Can you work these out from the model? Positions are in its coordinate system, mm. Face numbers are marked on the shaded views. A direction names the side the tool comes from. Coordinates: 2 decimals unless noted, no trailing zeros. Order: outer loops, then holes, each group sorted by start corner. A loop starts at its lowest first (then second) coordinate and runs counter-clockwise, first axis right, second up. Notation, with made-up numbers: (-3, 17) -> (38, 17) arc R12 ccw to (38, 25) -> close; hole circle Ø7 at (62.5, 6.25). An arc over 180 degrees is marked (long way). Answer as a JSON object with one key per item and string values. Group by question number.
(1) If we mould it in two halves opening along X, with no side actions, what happens to the marked faces 1, 2 and 3? For each: pulls with the +X half, pulls with the -X half, needs draft (parallel to the pull), parting line crosses it, or undercut.
(2) I want a section at C-C, the plane z = 8.5. List the corners of the cut face in (x, y) for me.
(3) For pin 1 (4.5 mm diameter, centred on y = 38.58, z = 7.34, fed in from -X); pin 2 (17.5 mm diameter, centred on x = 21.5, z = 24.5, fed in from +Y), each with a flat end and sliding along its axis, tell me the tip position at first contact or that it passes through.
(4) I need wall thicknesses on line 1 (Z direction, x = 20, y = 4); line 2 (X direction, y = 19, z = 19); line 3 (Z direction, x = 19.5, y = 4). Which ranges of each line are inside material? Lowest first, please.
(5) I want a section at D-D, the plane z = 28.5. List the corners of the cut face in (x, y) for me.
(6) Which directions (+Z, -Z, +X, -X, +Y, -Y) give clear straight access to the entire face, cutting with the end or side of a thin tool? Please do the marked faces 4 and 5.
(7) I want a section at A-A, the plane y = 12. List the corners of the cut face in (x, z) for me, plus the area to 3 significant figures.
(8) I want a section at B-B, the plane x = 20. List the corners of the cut face in (y, z) for me.
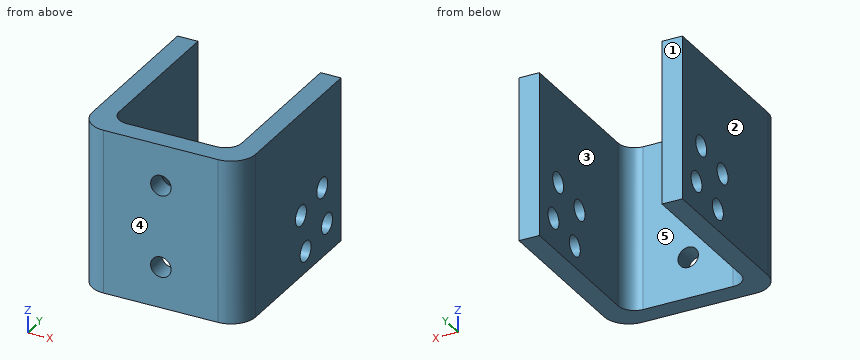
from build123d import *

# Parameters (mm, degrees)
RESSALTO_EXTRUS_O1_DEPTH = 40
FILETE1_R                = 6
ESBO_O3_R                = 2.5
CORTE_EXTRUS_O1_DEPTH    = 60
FILETE2_R                = 4
ESBO_O6_R                = 2.5
CORTE_EXTRUS_O4_DEPTH    = 5


with BuildPart() as part:
    # Esboço1 → Ressalto-extrusão1 (new body)
    with BuildSketch(Plane.XY):
        Polygon((0, 0), (0, 45), (5, 45), (5, 5), (35, 5), (35, 45), (40, 45), (40, 0), align=None)
    extrude(amount=RESSALTO_EXTRUS_O1_DEPTH)

    # Filete1
    filete1_edges = [part.edges().sort_by_distance(p)[0] for p in [
        (0, 0, 20),
        (40, 0, 20),
    ]]
    fillet(filete1_edges, radius=FILETE1_R)

    # Esboço3 → Corte-extrusão1 (cut)
    with BuildSketch(Plane.ZY):
        with Locations((7.342858474, 38.577006564)):
            Circle(ESBO_O3_R)
        with Locations((17.109227068, 36.428042981)):
            Circle(ESBO_O3_R)
        with Locations((14.960263485, 26.661674387)):
            Circle(ESBO_O3_R)
        with Locations((5.193894891, 28.810637969)):
            Circle(ESBO_O3_R)
    extrude(amount=-CORTE_EXTRUS_O1_DEPTH, mode=Mode.SUBTRACT)

    # Filete2
    filete2_edges = [part.edges().sort_by_distance(p)[0] for p in [
        (5, 5, 20),
        (35, 5, 20),
    ]]
    fillet(filete2_edges, radius=FILETE2_R)

    # Esboço6 → Corte-extrusão4 (cut)
    with BuildSketch(Plane.XZ):
        with Locations((20, 30)):
            Circle(ESBO_O6_R)
        with Locations((20, 10)):
            Circle(ESBO_O6_R)
    extrude(amount=-CORTE_EXTRUS_O4_DEPTH, mode=Mode.SUBTRACT)


solid = part.part
Computed values:
{
 "1": {"face 1": "needs draft", "face 2": "pulls with the -X half", "face 3": "undercut"},
 "2": {"outline": "(0, 6) arc R6 ccw to (6, 0) -> (18, 0) -> (18, 5) -> (9, 5) arc R4 cw to (5, 9) -> (5, 36.36) -> (0, 36.36) -> close; (0, 40.79) -> (5, 40.79) -> (5, 45) -> (0, 45) -> close; (22, 0) -> (34, 0) arc R6 ccw to (40, 6) -> (40, 36.36) -> (35, 36.36) -> (35, 9) arc R4 cw to (31, 5) -> (22, 5) -> close; (35, 40.79) -> (40, 40.79) -> (40, 45) -> (35, 45) -> close"},
 "3": {"pin 1": "passes through", "pin 2": "stops at y = 5"},
 "4": {"line 1": "z = 0 to 7.5, 12.5 to 27.5, 32.5 to 40", "line 2": "x = 0 to 5, 35 to 40", "line 3": "z = 0 to 7.55, 12.45 to 27.55, 32.45 to 40"},
 "5": {"outline": "(0, 6) arc R6 ccw to (6, 0) -> (18, 0) -> (18, 5) -> (9, 5) arc R4 cw to (5, 9) -> (5, 45) -> (0, 45) -> close; (22, 0) -> (34, 0) arc R6 ccw to (40, 6) -> (40, 45) -> (35, 45) -> (35, 9) arc R4 cw to (31, 5) -> (22, 5) -> close"},
 "6": {"face 4": "+Z, -Z, +X, -X, -Y", "face 5": "+Z, -Z, +Y"},
 "7": {"outline": "(0, 0) -> (5, 0) -> (5, 40) -> (0, 40) -> close; (35, 0) -> (40, 0) -> (40, 40) -> (35, 40) -> close", "area": "400 mm2"},
 "8": {"outline": "(0, 0) -> (5, 0) -> (5, 7.5) -> (0, 7.5) -> close; (0, 12.5) -> (5, 12.5) -> (5, 27.5) -> (0, 27.5) -> close; (0, 32.5) -> (5, 32.5) -> (5, 40) -> (0, 40) -> close"}
}
